```python
from build123d import *

# Parameters (mm, degrees)
BLANKSKE_W         = 210
BLANKSKE_H         = 6.5
BLANK_DEPTH        = 10
TOOTHCUTSIM_DEPTH  = 211.338417794
TEETHCUTS_COUNT    = 45
TEETHCUTS_PITCH    = 4.712388975
SKETCH1_R          = 1
SKETCH1_R_2        = 1.2
CUT_EXTRUDE1_DEPTH = 10


with BuildPart() as part:
    # BlankSke → Blank (new body)
    with BuildSketch(Plane.XY):
        with Locations((105, 3.25)):
            Rectangle(BLANKSKE_W, BLANKSKE_H)
    extrude(amount=-BLANK_DEPTH)

    # TooCutSkeSim → ToothCutSim (cut, through all)
    with BuildSketch(Plane.XY):
        Polygon((0.654653055, 3.125), (-0.654653055, 3.125), (-1.892297439, 6.5254), (1.892297439, 6.5254), align=None)
    toothcutsim = extrude(amount=-TOOTHCUTSIM_DEPTH, mode=Mode.SUBTRACT)

    # TeethCuts: ToothCutSim ×45
    with Locations(*[(i * TEETHCUTS_PITCH, 0, 0) for i in range(1, TEETHCUTS_COUNT)]):
        add(toothcutsim, mode=Mode.SUBTRACT)

    # Sketch1 → Cut-Extrude1 (cut)
    with BuildSketch(Plane(origin=(0, 0, -10), x_dir=(-1, 0, 0), z_dir=(0, 0, -1))):
        with Locations((-3.466384229, 1.5)):
            Circle(SKETCH1_R)
        with Locations((-198.448420537, 1.5)):
            Circle(SKETCH1_R_2)
        with Locations((-173.048420537, 1.5)):
            Circle(SKETCH1_R_2)
    extrude(amount=-CUT_EXTRUDE1_DEPTH, mode=Mode.SUBTRACT)


solid = part.part
```
Model file for the job. Use its own axes, mm. Give positions to 0.01 mm unless a question says otherwise; leave off trailing zeros. Write each loop counter-clockwise with the first axis right and the second up, starting at its lowest first coordinate (ties: lowest second). Pieces come first, ordered by that corner, then holes. Notation, with made-up numbers: (47, -35.5) - (106, -35.5) arc R20 ccw to (106, 3.5) - close; hole circle Ø3 at (52, 66.25). An arc over 180 degrees is marked (long way). One line per question, with ' | ' between items. Start each with the question number.
(1) Pin check, flat tip, straight feed: P1, Ø0.7, axis at x = 136.5, z = -6.5, coming from the +Y side (3 decimals). Stop position of the tip, or through.
(2) Two-plate mould, pull along X, no slides. Class faces 1 (the face through (189.773, 4.836, -4.93)), 2 (the face through (55.29, 4.79, -4.93)): +X half, -X half, draft (parallel to the pull), parting line (faces both ways), or undercut.
(3) Wall check: line 1 along X through (y, z) = (1.75, -8); line 2 along Y through (x, z) = (37.5, -4.5) (3 decimals). Give the ranges that are in metal, low to high. Write a range as from..to.
(4) Slice it at B-B on z = -7. Give the number of separate pieces and of enclosed holes in the cut face, plus the area to 3 significant figures.
(5) Slice it at A-A on y = 1.5. Write the cut outline in (x, z).
Results below:
1) P1: y = 3.125
2) face 1: undercut | face 2: undercut
3) line 1: 0..2.5, 4.43..171.87, 174.22..197.27, 199.62..210 | line 2: 0..3.125
4) separate pieces: 1 | enclosed holes: 3 | area: 972 mm^2
5) outline: (0, -10) - (2.47, -10) - (2.47, 0) - (0, 0) - close; (4.47, -10) - (171.85, -10) - (171.85, 0) - (4.47, 0) - close; (174.25, -10) - (197.25, -10) - (197.25, 0) - (174.25, 0) - close; (199.65, -10) - (210, -10) - (210, 0) - (199.65, 0) - close
